```python
from build123d import *

# Parameters (mm, degrees)
SKETCH_2_W           = 5
SKETCH_2_H           = 40
CUT_EXTRUDE_1_REACH  = 90.301
SKETCH_3_R           = 1.8
SKETCH_6_W           = 30
SKETCH_6_H           = 40
EXTRUDE_1_DEPTH      = 5
CUT_EXTRUDE_2_REACH  = 95.593
SKETCH_8_R           = 1.8
SKETCH_9_W           = 35
SKETCH_9_H           = 5
EXTRUDE_2_DEPTH      = 5
SKETCH_10_R          = 3.1
CUT_EXTRUDE_3_DEPTH  = 2
SKETCH_11_R          = 3.1
CUT_EXTRUDE_4_DEPTH  = 2
EXTRUDE_4_DEPTH      = 3
EXTRUDE_5_DEPTH      = 25
EXTRUDE_5_DEPTH_BACK = 25
CUT_EXTRUDE_5_REACH  = 150.427
SKETCH_17_R          = 1.8
SKETCH_18_R          = 3.5
CUT_EXTRUDE_6_DEPTH  = 3
EXTRUDE_6_DEPTH      = 34
RIB_4_REACH          = 156.717
SKETCH_20_WALL_W     = 374.245878862
SKETCH_20_WALL_H     = 5
RIB_5_REACH          = 156.717
SKETCH_21_WALL_W     = 340.795986182
SKETCH_21_WALL_H     = 5


with BuildPart() as part:
    # 扫描1: sweep along a path in 草图1
    with BuildLine(Plane.XY) as sweep_1_path:
        Line((0, 0), (0, 45))
        Line((0, 45), (14.36484602, 84.467090073))
    # 草图2 → 扫描1 (sweep)
    with BuildSketch(Plane(origin=(0, 0, 0), x_dir=(1, 0, 0), z_dir=(0, 1, 0))):
        with Locations((2.5, 0)):
            Rectangle(SKETCH_2_W, SKETCH_2_H)
    sweep(path=sweep_1_path.line, transition=Transition.RIGHT)

    # 草图3 → 切除-拉伸1 (cut, up to next)
    with BuildSketch(Plane(origin=(-14.462721218, 5.26400003, 0), x_dir=(0, 0, 1), z_dir=(-0.9396926207859081, 0.3420201433256695, 0)), mode=Mode.PRIVATE) as cut_extrude_1_sk1:
        with Locations(Location((-10, 66.286167935, 0), (0, 0, 270))):
            Circle(SKETCH_3_R)
    cut_extrude_1_tool1 = extrude(cut_extrude_1_sk1.sketch, amount=-CUT_EXTRUDE_1_REACH, mode=Mode.PRIVATE) & part.part
    # 草图3 → 切除-拉伸1 (cut, up to next)
    with BuildSketch(Plane(origin=(-14.462721218, 5.26400003, 0), x_dir=(0, 0, 1), z_dir=(-0.9396926207859081, 0.3420201433256695, 0)), mode=Mode.PRIVATE) as cut_extrude_1_sk2:
        with Locations(Location((10, 66.286167935, 0), (0, 0, 270))):
            Circle(SKETCH_3_R)
    cut_extrude_1_tool2 = extrude(cut_extrude_1_sk2.sketch, amount=-CUT_EXTRUDE_1_REACH, mode=Mode.PRIVATE) & part.part
    add(cut_extrude_1_tool1.solids().sort_by_distance((8.208483, 67.552623, -10))[0], mode=Mode.SUBTRACT)
    add(cut_extrude_1_tool2.solids().sort_by_distance((8.208483, 67.552623, 10))[0], mode=Mode.SUBTRACT)

    # 草图6 → 凸台-拉伸1 (add)
    with BuildSketch(Plane.XZ):
        with Locations((20, 0)):
            Rectangle(SKETCH_6_W, SKETCH_6_H)
    extrude(amount=-EXTRUDE_1_DEPTH)

    # 草图8 → 切除-拉伸2 (cut, up to next)
    with BuildSketch(Plane.XZ, mode=Mode.PRIVATE) as cut_extrude_2_sk1:
        with Locations(Location((10, 17.5, 0), (0, 0, 270))):
            Circle(SKETCH_8_R)
    cut_extrude_2_tool1 = extrude(cut_extrude_2_sk1.sketch, amount=-CUT_EXTRUDE_2_REACH, mode=Mode.PRIVATE) & part.part
    # 草图8 → 切除-拉伸2 (cut, up to next)
    with BuildSketch(Plane.XZ, mode=Mode.PRIVATE) as cut_extrude_2_sk2:
        with Locations(Location((10, -17.5, 0), (0, 0, 270))):
            Circle(SKETCH_8_R)
    cut_extrude_2_tool2 = extrude(cut_extrude_2_sk2.sketch, amount=-CUT_EXTRUDE_2_REACH, mode=Mode.PRIVATE) & part.part
    # 草图8 → 切除-拉伸2 (cut, up to next)
    with BuildSketch(Plane.XZ, mode=Mode.PRIVATE) as cut_extrude_2_sk3:
        with Locations(Location((30, 0, 0), (0, 0, 270))):
            Circle(SKETCH_8_R)
    cut_extrude_2_tool3 = extrude(cut_extrude_2_sk3.sketch, amount=-CUT_EXTRUDE_2_REACH, mode=Mode.PRIVATE) & part.part
    add(cut_extrude_2_tool1.solids().sort_by_distance((10, 0, 17.5))[0], mode=Mode.SUBTRACT)
    add(cut_extrude_2_tool2.solids().sort_by_distance((10, 0, -17.5))[0], mode=Mode.SUBTRACT)
    add(cut_extrude_2_tool3.solids().sort_by_distance((30, 0, 0))[0], mode=Mode.SUBTRACT)

    # 草图9 → 凸台-拉伸2 (add)
    with BuildSketch(Plane.XZ):
        with Locations((17.5, 22.5)):
            Rectangle(SKETCH_9_W, SKETCH_9_H)
        with Locations((17.5, -22.5)):
            Rectangle(SKETCH_9_W, SKETCH_9_H)
    extrude(amount=-EXTRUDE_2_DEPTH)

    # 草图10 → 切除-拉伸3 (cut)
    with BuildSketch(Plane(origin=(0, 5, 0), x_dir=(1, 0, 0), z_dir=(0, 1, 0))):
        with Locations(Location((10, -17.5, 0), (0, 0, 270))):
            Circle(SKETCH_10_R)
        with Locations(Location((10, 17.5, 0), (0, 0, 270))):
            Circle(SKETCH_10_R)
        with Locations(Location((30, 0, 0), (0, 0, 270))):
            Circle(SKETCH_10_R)
    extrude(amount=-CUT_EXTRUDE_3_DEPTH, mode=Mode.SUBTRACT)

    # 草图11 → 切除-拉伸4 (cut)
    with BuildSketch(Plane(origin=(-14.462721218, 5.26400003, 0), x_dir=(0, 0, 1), z_dir=(-0.9396926207859081, 0.3420201433256695, 0))):
        with Locations(Location((-10, 66.286167935, 0), (0, 0, 270))):
            Circle(SKETCH_11_R)
        with Locations(Location((10, 66.286167935, 0), (0, 0, 270))):
            Circle(SKETCH_11_R)
    extrude(amount=-CUT_EXTRUDE_4_DEPTH, mode=Mode.SUBTRACT)

    # 草图15 → 凸台-拉伸4 (add)
    with BuildSketch(Plane(origin=(0, 0, -20), x_dir=(-1, 0, 0), z_dir=(0, 0, -1))):
        Polygon((-8.680805733, 84.407556003), (-13.680805733, 82.587704831), (0, 45), (0, 5), (10, 5), (10, 84.407556003), align=None)
    extrude_4 = extrude(amount=-EXTRUDE_4_DEPTH)

    # 镜向2: 凸台-拉伸4 across plane
    add(extrude_4.mirror(Plane(origin=(0, 0, 0), x_dir=(1, 0, 0), z_dir=(0, 0, -1))))

    # 草图16 → 凸台-拉伸5 (add, two sides: drawn at the far end of the back side and taken through both)
    with BuildSketch(Plane(origin=(0, 0, 0), x_dir=(-1, 0, 0), z_dir=(0, 0, -1)).offset(-EXTRUDE_5_DEPTH_BACK)):
        Polygon((-14.36484602, 84.467090073), (2.824266896, 148.61773281), (8.142432199, 147.192734712), (-8.680805733, 84.407556003), (-13.680805733, 82.587704831), align=None)
    extrude(amount=EXTRUDE_5_DEPTH + EXTRUDE_5_DEPTH_BACK)

    # 草图17 → 切除-拉伸5 (cut, up to next)
    with BuildSketch(Plane(origin=(34.519356315, 9.249433648, 0), x_dir=(0, 0, -1), z_dir=(0.9659258262890672, 0.2588190451025248, 0)), mode=Mode.PRIVATE) as cut_extrude_5_sk1:
        with Locations(Location((-18, 134.371048043, 0), (0, 0, 90))):
            Circle(SKETCH_17_R)
    cut_extrude_5_tool1 = extrude(cut_extrude_5_sk1.sketch, amount=-CUT_EXTRUDE_5_REACH, mode=Mode.PRIVATE) & part.part
    # 草图17 → 切除-拉伸5 (cut, up to next)
    with BuildSketch(Plane(origin=(34.519356315, 9.249433648, 0), x_dir=(0, 0, -1), z_dir=(0.9659258262890672, 0.2588190451025248, 0)), mode=Mode.PRIVATE) as cut_extrude_5_sk2:
        with Locations(Location((18, 134.371048043, 0), (0, 0, 90))):
            Circle(SKETCH_17_R)
    cut_extrude_5_tool2 = extrude(cut_extrude_5_sk2.sketch, amount=-CUT_EXTRUDE_5_REACH, mode=Mode.PRIVATE) & part.part
    # 草图17 → 切除-拉伸5 (cut, up to next)
    with BuildSketch(Plane(origin=(34.519356315, 9.249433648, 0), x_dir=(0, 0, -1), z_dir=(0.9659258262890672, 0.2588190451025248, 0)), mode=Mode.PRIVATE) as cut_extrude_5_sk3:
        with Locations(Location((18, 86.371048043, 0), (0, 0, 90))):
            Circle(SKETCH_17_R)
    cut_extrude_5_tool3 = extrude(cut_extrude_5_sk3.sketch, amount=-CUT_EXTRUDE_5_REACH, mode=Mode.PRIVATE) & part.part
    # 草图17 → 切除-拉伸5 (cut, up to next)
    with BuildSketch(Plane(origin=(34.519356315, 9.249433648, 0), x_dir=(0, 0, -1), z_dir=(0.9659258262890672, 0.2588190451025248, 0)), mode=Mode.PRIVATE) as cut_extrude_5_sk4:
        with Locations(Location((-18, 86.371048043, 0), (0, 0, 90))):
            Circle(SKETCH_17_R)
    cut_extrude_5_tool4 = extrude(cut_extrude_5_sk4.sketch, amount=-CUT_EXTRUDE_5_REACH, mode=Mode.PRIVATE) & part.part
    add(cut_extrude_5_tool1.solids().sort_by_distance((-0.25843, 139.041899, 18))[0], mode=Mode.SUBTRACT)
    add(cut_extrude_5_tool2.solids().sort_by_distance((-0.25843, 139.041899, -18))[0], mode=Mode.SUBTRACT)
    add(cut_extrude_5_tool3.solids().sort_by_distance((12.164884, 92.67746, -18))[0], mode=Mode.SUBTRACT)
    add(cut_extrude_5_tool4.solids().sort_by_distance((12.164884, 92.67746, 18))[0], mode=Mode.SUBTRACT)

    # 草图18 → 切除-拉伸6 (cut)
    with BuildSketch(Plane(origin=(29.201191012, 7.82443555, 0), x_dir=(0, 0, 1), z_dir=(-0.9659258262890674, -0.2588190451025246, 0))):
        with Locations(Location((-18, 134.371048043, 0), (0, 0, 270))):
            Circle(SKETCH_18_R)
        with Locations(Location((18, 134.371048043, 0), (0, 0, 270))):
            Circle(SKETCH_18_R)
        with Locations(Location((18, 86.371048043, 0), (0, 0, 270))):
            Circle(SKETCH_18_R)
        with Locations(Location((-18, 86.371048043, 0), (0, 0, 270))):
            Circle(SKETCH_18_R)
    extrude(amount=-CUT_EXTRUDE_6_DEPTH, mode=Mode.SUBTRACT)

    # 草图19 → 凸台-拉伸6 (add)
    with BuildSketch(Plane.XY.offset(-17)):
        Polygon((12.654745303, 79.768626969), (8.151824791, 81.407556003), (-10, 81.407556003), (-10, 84.407556003), (8.680805733, 84.407556003), (13.680805733, 82.587704831), align=None)
    extrude(amount=EXTRUDE_6_DEPTH)

    # 草图20 wall → 筋4 (add, up to next)
    with BuildSketch(Plane(origin=(-9.071216099, 115.800145357, 0), x_dir=(0.029573147262, 0.999562618829, 0), z_dir=(0.999562618829, -0.029573147262, 0)), mode=Mode.PRIVATE) as rib_4_sk1:
        Rectangle(SKETCH_20_WALL_W, SKETCH_20_WALL_H)
    rib_4_tool1 = extrude(rib_4_sk1.sketch, amount=RIB_4_REACH, mode=Mode.PRIVATE) - part.part
    add(rib_4_tool1.solids().sort_by_distance((-9.071216099, 115.800145357, 0))[0])

    # 草图21 wall → 筋5 (add, up to next)
    with BuildSketch(Plane(origin=(15.95, 14.779591274, 0), x_dir=(0.745842716131, -0.666122093009, 0), z_dir=(-0.666122093009, -0.745842716131, 0)), mode=Mode.PRIVATE) as rib_5_sk1:
        Rectangle(SKETCH_21_WALL_W, SKETCH_21_WALL_H)
    rib_5_tool1 = extrude(rib_5_sk1.sketch, amount=RIB_5_REACH, mode=Mode.PRIVATE) - part.part
    add(rib_5_tool1.solids().sort_by_distance((15.95, 14.779591274, 0))[0])


solid = part.part
```
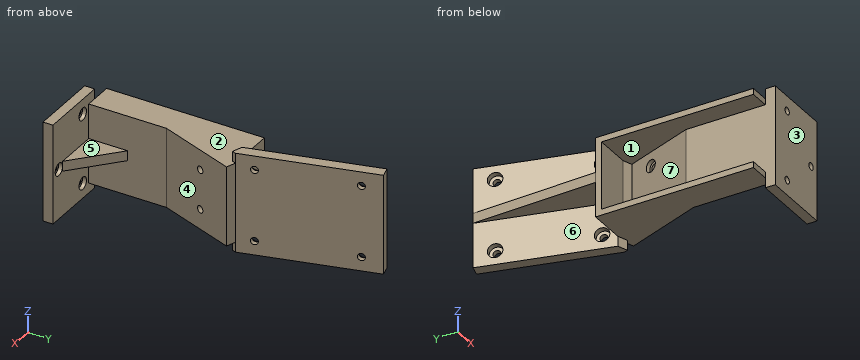
Read the model definition and answer for the solid it produces. Units are mm, in the model's axes. Face numbers are marked on the shaded views. A direction names the side the tool comes from. Coordinates: 2 decimals unless noted, no trailing zeros. Write each loop counter-clockwise with the first axis right and the second up, starting at its lowest first coordinate (ties: lowest second). Pieces come first, ordered by that corner, then holes. Notation, with made-up numbers: (-13.75, 60) - (3.25, 60) arc R20 ccw to (3.25, 93) - close; hole circle Ø1 at (53.5, 80.25). An arc over 180 degrees is marked (long way). Answer as a JSON object with one key per item and string values. Group by question number.
1. A cutting plane is placed at B-B (y = 34). Determine the outline of the cut face in (x, z), plus the area to 3 significant figures.
2. The mould has two halves that part along Z. Classify the marked faces 1, 2 and 3: +Z half, -Z half, draft (parallel to the pull), parting line (faces both ways), or undercut.
3. Which of the six approach directions +Z, -Z, +X, -X, +Y, -Y give full straight-line access (tool end or side, diameter ignored) to the marked faces 4, 5, 6 and 7?
4. Each of these flat-tipped pins is pushed along its axis until it touches: P1, Ø2, axis at y = 91, z = 8, coming from the +X side; P2, Ø18, axis at x = -1.5, y = 56, coming from the -Z side; P3, Ø5, axis at x = 29.5, z = -1.5, coming from the +Y side. Where does it stop, or does it pass through?
5. A cutting plane is placed at C-C (x = 25). Determine the outline of the cut face in (y, z), plus the area to 3 significant figures.
6. Consider L1, parallel to X at y = 2, z = 0; L2, parallel to Z at x = -4, y = 11; L3, parallel to Y at x = 33, z = 20. Determine where each line is inside the solid, lowest interval first. Write a range as [from, to].
7. A cutting plane is placed at A-A (x = 16). Determine the outline of the cut face in (y, z).
Worked out:
{
 "1": {"outline": "(-10, -20) - (5, -20) - (5, 20) - (-10, 20) - (-10, 17) - (0, 17) - (0, -17) - (-10, -17) - close", "area": "260 mm²"},
 "2": {"face 1": "undercut", "face 2": "+Z half", "face 3": "draft"},
 "3": {"face 4": "+Z, -Z, +X", "face 5": "+Z, +X", "face 6": "-Z, -X", "face 7": "-X"},
 "4": {"P1": "stops at x = 12.88", "P2": "stops at z = -20", "P3": "stops at y = 5"},
 "5": {"outline": "(0, -25) - (5, -25) - (5, -2.5) - (6.7, -2.5) - (6.7, 2.5) - (5, 2.5) - (5, 25) - (0, 25) - close", "area": "258 mm²"},
 "6": {"L1": "x = [0, 28.2], [31.8, 35]", "L2": "z = [-20, -17], [17, 20]", "L3": "y = [0, 5]"},
 "7": {"outline": "(0, -25) - (5, -25) - (5, -2.5) - (14.73, -2.5) - (14.73, 2.5) - (5, 2.5) - (5, 25) - (0, 25) - close; (74.34, -20) - (83.87, -20) - (83.87, 20) - (74.34, 20) - close"}
}
